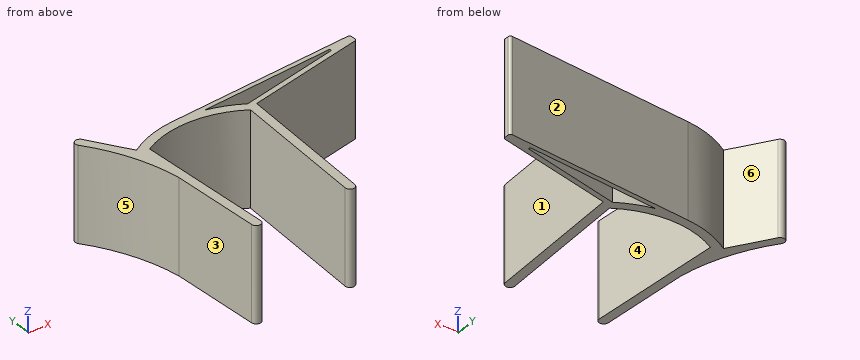
from build123d import *

# Parameters (mm, degrees)
F1_DEPTH = 20


with BuildPart() as f1:
    # F0 (on Top) → F1 (new body)
    with BuildSketch(Plane.XY):
        with BuildLine():
            ThreePointArc((-10.407943, -26.715306), (-9.351406, -27.655374), (-8.411337, -26.598837))
            Line((-8.411337, -26.598837), (-10.407943, -26.715306))
        make_face()
        with BuildLine():
            Line((11.585269, -26.715306), (9.588663, -26.598837))
            ThreePointArc((9.588663, -26.598837), (10.528732, -27.655374), (11.585269, -26.715306))
        make_face()
        with BuildLine():
            ThreePointArc((-10.161337, 3.401163), (0.588663, 6.401163), (11.338663, 3.401163))
            Line((11.338663, 3.401163), (9.588663, -26.598837))
            Line((9.588663, -26.598837), (11.585269, -26.715306))
            Line((11.585269, -26.715306), (13.400839, 4.40875))
            ThreePointArc((13.400839, 4.40875), (12.751886, 4.835248), (12.08875, 5.23934))
            ThreePointArc((12.08875, 5.23934), (8.584038, 6.909612), (4.846286, 7.959386))
            ThreePointArc((4.846286, 7.959386), (1.485483, 8.343819), (-1.895165, 8.225455))
            ThreePointArc((-1.895165, 8.225455), (-7.293833, 6.951665), (-12.223513, 4.40875))
            Line((-12.223513, 4.40875), (-11.555542, -7.042185))
            Line((-11.555542, -7.042185), (-10.407943, -26.715306))
            Line((-10.407943, -26.715306), (-8.411337, -26.598837))
            Line((-8.411337, -26.598837), (-10.161337, 3.401163))
        make_face()
        with BuildLine():
            ThreePointArc((-19.390229, 11.663968), (-14.25265, 2.821962), (-11.555542, -7.042185))
            Line((-11.555542, -7.042185), (-12.223513, 4.40875))
            Line((-12.223513, 4.40875), (-17.719352, 12.763136))
            Line((-17.719352, 12.763136), (-19.390229, 11.663968))
        make_face()
        with BuildLine():
            ThreePointArc((-17.719352, 12.763136), (-19.104374, 13.04899), (-19.390229, 11.663968))
            Line((-19.390229, 11.663968), (-17.719352, 12.763136))
        make_face()
        with BuildLine():
            ThreePointArc((12.08875, 5.23934), (12.751886, 4.835248), (13.400839, 4.40875))
            Line((13.400839, 4.40875), (39.021619, 10.786566))
            ThreePointArc((39.021619, 10.786566), (39.294787, 10.963855), (39.400839, 11.271759))
            Line((39.400839, 11.271759), (39.400839, 12.205185))
            ThreePointArc((39.400839, 12.205185), (39.234526, 12.577547), (38.846227, 12.702194))
            Line((38.846227, 12.702194), (-1.895165, 8.225455))
            ThreePointArc((-1.895165, 8.225455), (1.485483, 8.343819), (4.846286, 7.959386))
            Line((4.846286, 7.959386), (33.684866, 11.128222))
            ThreePointArc((33.684866, 11.128222), (33.958279, 10.923665), (33.772562, 10.637121))
            Line((33.772562, 10.637121), (12.08875, 5.23934))
        make_face()
    extrude(amount=F1_DEPTH)


solid = f1.part
Design review of the part built by this model. Coordinates are the model's own, in mm. Face numbers are marked on the shaded views. A direction names the side the tool comes from. Give positions to 0.01 mm unless a question says otherwise; leave off trailing zeros. Write each loop counter-clockwise with the first axis right and the second up, starting at its lowest first coordinate (ties: lowest second). Pieces come first, ordered by that corner, then holes. Notation, with made-up numbers: M -12,37.5 L 14,37.5 A13 cw 14,47.5 Z; hole C 61,-17.75 d7. An arc over 180 degrees is marked long. Return JSON: item names as keys, results as strings. Group by question number.
Item 1: Take a section at D-D (x = 14.5). Give the boundary of the cut face in (y, z).
Item 2: Take a section at C-C (y = 9.5). Give the boundary of the cut face in (x, z).
Item 3: Take a section at B-B (z = 8). Give the boundary of the cut face in (x, y), plus the area to 3 significant figures.
Item 4: Clearance check with flat-ended pins moving along their axes: pin 1 Ø2 at (y, z) = (3, 7.5) entering from -X; pin 2 Ø3 at (y, z) = (-3.5, 15.5) entering from -X; pin 3 Ø3 at (y, z) = (-10.5, 11.5) entering from +X. State where each tip first meets the part, or that it passes through.
Item 5: Tool access review of the marked faces 4, 5 and 6: name each direction out of +Z, -Z, +X, -X, +Y, -Y from which nothing blocks a thin tool from reaching the whole face with its end or side.
Item 6: The part is to be moulded in two halves that separate along X. For the marked faces 1, 2 and 3, say which applies: pulls with the +X half, pulls with the -X half, needs draft (parallel to the pull), parting line crosses it, or undercut.
Item 7: Take a section at A-A (y = -21). Give the boundary of the cut face in (x, z), plus the area to 3 significant figures.
Item 8: Wall thickness on line 1 along X through (y, z) = (-6, 12.5); line 2 along Y through (x, z) = (32.5, 10.5); line 3 along X through (y, z) = (-13, 9.25): over which ranges is each line inside the solid? List them lowest first.
Return value:
{
 "1": {"outline": "M 4.68,0 L 5.84,0 L 5.84,20 L 4.68,20 Z; M 9.02,0 L 10.03,0 L 10.03,20 L 9.02,20 Z"},
 "2": {"outline": "M -17.84,0 L -15.57,0 L -15.57,20 L -17.84,20 Z; M 9.7,0 L 18.87,0 L 18.87,20 L 9.7,20 Z; M 29.2,0 L 33.85,0 L 33.85,20 L 29.2,20 Z"},
 "3": {"outline": "M -19.39,11.66 A39.52 cw -11.56,-7.04 L -10.41,-26.72 A1 ccw -8.41,-26.6 L -10.16,3.4 A20.76 cw 11.34,3.4 L 9.59,-26.6 A1 ccw 11.59,-26.72 L 13.4,4.41 L 39.02,10.79 A0.5 ccw 39.4,11.27 L 39.4,12.21 A0.5 ccw 38.85,12.7 L -1.9,8.23 A22.74 ccw -12.22,4.41 L -17.72,12.76 A1 ccw Z; hole M 4.85,7.96 A22.74 cw 12.09,5.24 L 33.77,10.64 A0.25 ccw 33.68,11.13 Z", "area": "275 mm2"},
 "4": {"pin 1": "stops at x = -14.77", "pin 2": "stops at x = -12.59", "pin 3": "stops at x = 12.62"},
 "5": {"face 4": "+Z, -Z", "face 5": "+Z, -Z, -X, -Y", "face 6": "+Z, -Z, +Y"},
 "6": {"face 1": "pulls with the +X half", "face 2": "undercut", "face 3": "pulls with the -X half"},
 "7": {"outline": "M -10.74,0 L -8.74,0 L -8.74,20 L -10.74,20 Z; M 9.92,0 L 11.92,0 L 11.92,20 L 9.92,20 Z", "area": "80.1 mm2"},
 "8": {"line 1": "x = -11.71 to -9.61, 10.79 to 12.79", "line 2": "y = 9.16 to 10.32, 11 to 12", "line 3": "x = -11.21 to -9.2, 10.38 to 12.39"}
}
